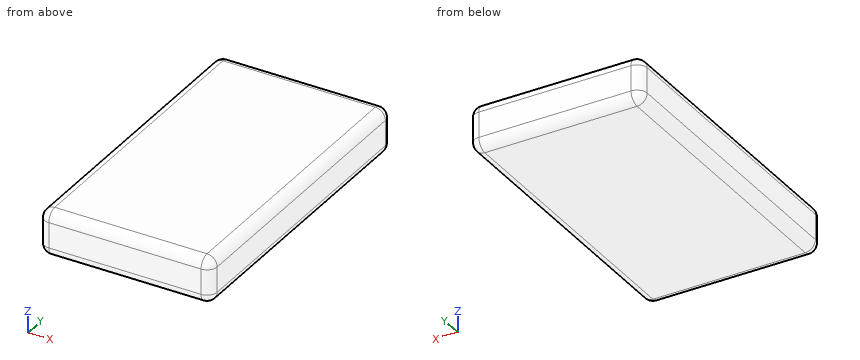
Solid Edge part; units mm, degrees
sketch "Sketch1" plane through (0, 0, 0) normal (0, 0, 1) x (1, 0, 0)
  line L0 (0.7047, -78.9141) -> (34.7047, -78.9141)
  line L1 (34.7047, -78.9141) -> (34.7047, -18.9141)
  line L2 (34.7047, -18.9141) -> (0.7047, -18.9141)
  line L3 (0.7047, -18.9141) -> (0.7047, -78.9141)
extrude "Protrusion1" add sketch "Sketch1" along normal blind 9
fillet "Round_1" radius 2 12 edges at (0.7047, -48.9141, 0) (17.7047, -78.9141, 0) (34.7047, -48.9141, 0) (17.7047, -18.9141, 0) (34.7047, -48.9141, 9) (17.7047, -78.9141, 9) (0.7047, -48.9141, 9) (17.7047, -18.9141, 9) (0.7047, -18.9141, 4.5) (0.7047, -78.9141, 4.5) (34.7047, -78.9141, 4.5) (34.7047, -18.9141, 4.5)
properties material "Zinc"
For this review, take the finished solid that the model builds, in its own axes (mm). Round coordinates to 2 decimals unless told otherwise and drop trailing zeros. Loops run counter-clockwise (first coordinate to the right, second up) from the corner with the lowest first, then second, coordinate; pieces in that order, holes last. Notation, with made-up numbers: (-16, 53) - (13, 53) arc R12 ccw to (13, 70) - close; hole circle Ø10 at (23, 72). An arc over 180 degrees is marked (long way). One line per question, with ' | ' between items.
Q1. For pin 1 (10 mm diameter, centred on x = 25.5, y = -66.5, fed in from -Z), flat-tipped, find the tip position at first contact; note if it passes through.
Taken from the geometry:
pin 1: stops at z = 0
Q2. Take a section at A-A (z = 8.25). Give the boundary of the cut face in (x, y), and give its area (3 significant figures).
Taken from the geometry:
outline: (1.14, -76.91) arc R1.56 ccw to (2.7, -78.48) - (32.7, -78.48) arc R1.56 ccw to (34.27, -76.91) - (34.27, -20.91) arc R1.56 ccw to (32.7, -19.35) - (2.7, -19.35) arc R1.56 ccw to (1.14, -20.91) - close | area: 1,960 mm²
Q3. For line 1 along Y through (x, z) = (22.5, 1.25); line 2 along Y through (x, z) = (30.5, 1); line 3 along X through (y, z) = (-71.5, 8), list the stretches that pass through material, from the lowest coordinate up. Write a range as [from, to].
Taken from the geometry:
line 1: y = [-78.77, -19.06] | line 2: y = [-78.65, -19.18] | line 3: x = [0.97, 34.44]
